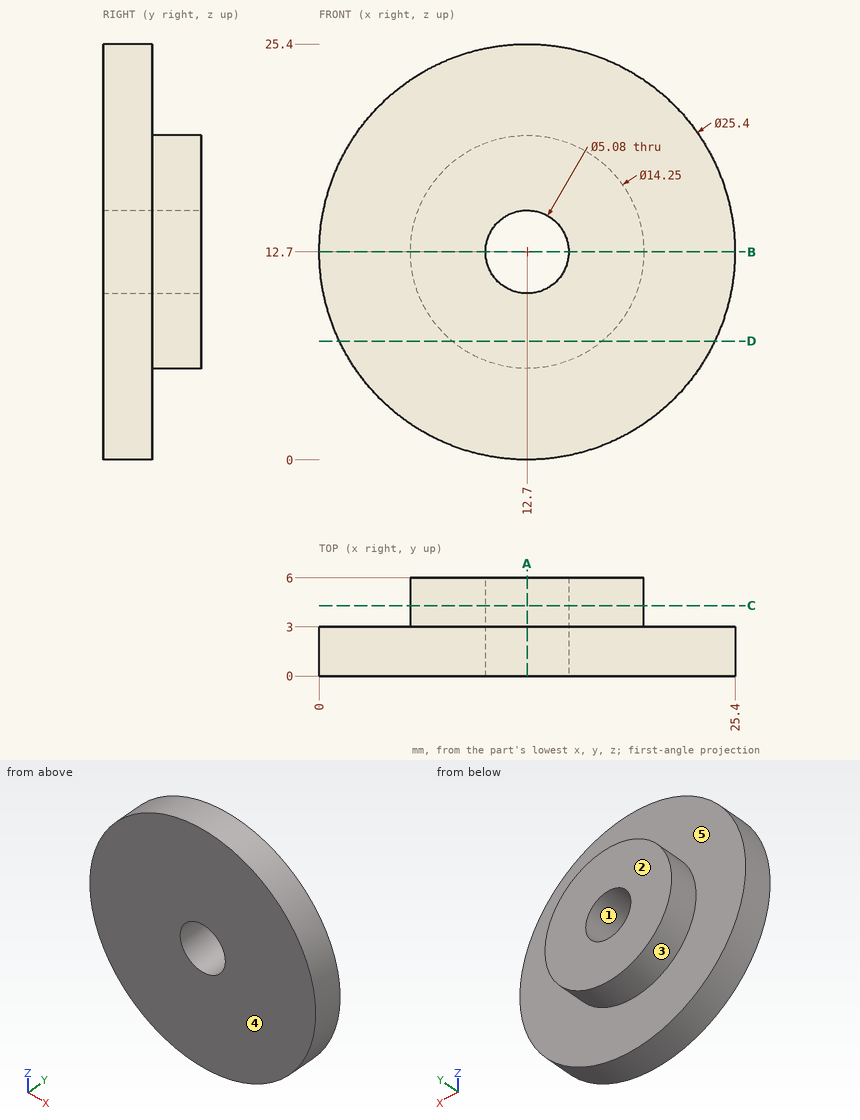
Here's the drawing with two shaded views (mm, measured from the low corner). I have some questions. A direction names the side the tool comes from. Round coordinates to 2 decimals unless told otherwise and drop trailing zeros. Loops run counter-clockwise (first coordinate to the right, second up) from the corner with the lowest first, then second, coordinate; pieces in that order, holes last.
Item 1: Suppose I cut it at C-C, the plane y = 4.3. Write out the boundary of the cut face in (x, z) (3 decimals), then the cut area to 3 significant figures.
Item 2: Which directions (+Z, -Z, +X, -X, +Y, -Y) give clear straight access to the entire face, cutting with the end or side of a thin tool? Please do the marked faces 4 and 5.
Item 3: If we mould it in two halves opening along Z, with no side actions, what happens to the marked faces 1, 2 and 3? For each: +Z half, -Z half, draft (parallel to the pull), parting line (faces both ways), or undercut.
Item 4: Suppose I cut it at D-D, the plane z = 7.25. Write out the boundary of the cut face in (x, y), then the cut area to 3 significant figures.
Item 5: Suppose I cut it at B-B, the plane z = 12.7. Write out the boundary of the cut face in (x, y) (3 decimals), then the cut area to 3 significant figures.
Item 6: Suppose I cut it at A-A, the plane x = 12.7. Write out the boundary of the cut face in (y, z) (3 decimals), then the cut area to 3 significant figures.
Item 7: Will these pins go through, and if not, where does the flat tip stop? pin 1 Ø3 at (x, y) = (19.5, 0.5) entering from +Z; pin 2 Ø3 at (y, z) = (3.5, 10.5) entering from +X; pin 3 Ø3 at (x, y) = (9, 5) entering from +Z.
Item 8: Please list where these lines run through material, in increasing order: L1, parallel to Z at x = 12.7, y = 3.1 (3 decimals); L2, parallel to Y at x = 14.5, z = 3.
Reported:
1. outline: circle Ø14.25 at (12.7, 12.7); hole circle Ø5.08 at (12.7, 12.7)
1. area: 139 mm2
2. face 4: +Z, -Z, +X, -X, -Y
2. face 5: +Y
3. face 1: undercut
3. face 2: draft
3. face 3: parting line
4. outline: (1.23, 0) - (24.17, 0) - (24.17, 3) - (17.29, 3) - (17.29, 6) - (8.11, 6) - (8.11, 3) - (1.23, 3) - close
4. area: 96.4 mm2
5. outline: (0, 0) - (10.16, 0) - (10.16, 6) - (5.575, 6) - (5.575, 3) - (0, 3) - close; (15.24, 0) - (25.4, 0) - (25.4, 3) - (19.825, 3) - (19.825, 6) - (15.24, 6) - close
5. area: 88.5 mm2
6. outline: (0, 0) - (3, 0) - (3, 5.575) - (6, 5.575) - (6, 10.16) - (0, 10.16) - close; (0, 15.24) - (6, 15.24) - (6, 19.825) - (3, 19.825) - (3, 25.4) - (0, 25.4) - close
6. area: 88.5 mm2
7. pin 1: stops at z = 24.24
7. pin 2: stops at x = 25.38
7. pin 3: stops at z = 19.48
8. L1: z = 5.575 to 10.16, 15.24 to 19.825
8. L2: y = 0 to 3
